Read the model definition and answer for the solid it produces. Units are mm, in the model's axes. Coordinates: 2 decimals unless noted, no trailing zeros. Write each loop counter-clockwise with the first axis right and the second up, starting at its lowest first coordinate (ties: lowest second). Pieces come first, ordered by that corner, then holes. Notation, with made-up numbers: M 58,74 L 83,74 A17 ccw 83,101 Z; hole C 18,54 d9. An arc over 180 degrees is marked long. Write item = value, one per line.
from build123d import *

# Parameters (mm, degrees)
F0_R     = 3.5
F0_W     = 13
F0_H     = 10
F1_DEPTH = 1.5


with BuildPart() as f1:
    # F0 (on Front) → F1 (new body, symmetric)
    with BuildSketch(Plane.XZ):
        Polygon((-29.5, -13), (29.5, -13), (29.5, 13), (20.5, 13), (7.5, 13), (-7.5, 13), (-20.5, 13), (-29.5, 13), align=None)
        with Locations((0, -7.445684)):
            Circle(F0_R, mode=Mode.SUBTRACT)
        with Locations((-14.590251, 6.649186)):
            Circle(F0_R, mode=Mode.SUBTRACT)
        with Locations((14.393566, 7.443263)):
            Circle(F0_R, mode=Mode.SUBTRACT)
        with Locations((14, 18)):
            Rectangle(F0_W, F0_H)
        with Locations((-14, 18)):
            Rectangle(F0_W, F0_H)
    extrude(amount=F1_DEPTH, both=True)


solid = f1.part
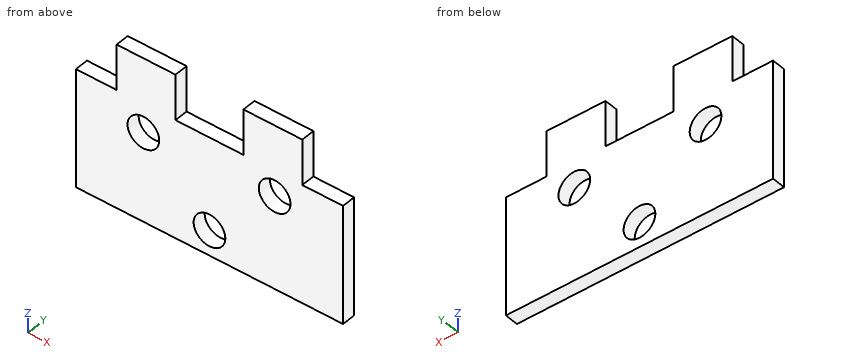
Item 1: Find section B-B (y = 0.45). Determine the outline of the cut face in (x, z).
Worked answers:
outline = M -29.5,-13 L 29.5,-13 L 29.5,13 L 20.5,13 L 20.5,23 L 7.5,23 L 7.5,13 L -7.5,13 L -7.5,23 L -20.5,23 L -20.5,13 L -29.5,13 Z; hole C -14.59,6.65 d7; hole C 0,-7.45 d7; hole C 14.39,7.44 d7
Item 2: Consider line 1 along Z through (x, y) = (0, -0.1); line 2 along X through (y, z) = (-0.5, 15); line 3 along X through (y, z) = (-0.65, 9). Determine where each line is inside the solid, lowest interval first. Write a range as from..to.
Worked answers:
line_1 = -13..-10.95, -3.95..13
line_2 = -20.5..-7.5, 7.5..20.5
line_3 = -29.5..-17.18, -12..11.26, 17.53..29.5
Item 3: Find section A-A (x = 0). Determine the outline of the cut face in (y, z).
Worked answers:
outline = M -1.5,-13 L 1.5,-13 L 1.5,-10.95 L -1.5,-10.95 Z; M -1.5,-3.95 L 1.5,-3.95 L 1.5,13 L -1.5,13 Z
Item 4: Flat-ended cylindrical pins translate along their axes: pin 1 (0.9 mm diameter, centred on x = 24, y = 0, fed in from +Z); pin 2 (5.5 mm diameter, centred on x = 0, z = -7.45, fed in from -Y). Find the tip coordinate at first contact, or state that the pin passes through.
Worked answers:
pin_1 = 13
pin_2 = through
Item 5: Find section C-C (x = -24). Determine the outline of the cut face in (y, z).
Worked answers:
outline = M -1.5,-13 L 1.5,-13 L 1.5,13 L -1.5,13 Z
